The model under review builds one solid part; all positions refer to its coordinate system, in mm. A direction names the side the tool comes from. Coordinates: 2 decimals unless noted, no trailing zeros. Write each loop counter-clockwise with the first axis right and the second up, starting at its lowest first coordinate (ties: lowest second). Pieces come first, ordered by that corner, then holes.
1) Mouldability with a two-part tool opening along X and no side actions: class faces 1 (the flat face through (0, 7.485, 1)), 2 (the flat face through (5.047, 6, 1)), 3 (the cylindrical face through (120, 0, 1)), 4 (the flat face through (54, 0, 3)) as released by +X, released by -X, zero draft, split by the parting line, or undercut.
2) Add section D-D, the plane x = 2.5. State the section outline as (y, z) points.
3) Machinability: for faces 5 (the flat face through (0, 4.985, 1)), 6 (the flat face through (54, -10, 1)), which of the approach directions +Z, -Z, +X, -X, +Y, -Y give a long, thin tool a straight path to every point of the face, cutting with its end or side? Answer none if there is none.
4) Add section A-A, the plane x = 20. State the section outline as (y, z) points.
5) For line 1 (Y direction, x = 0, z = 0.75); line 2 (Y direction, x = 110, z = 2.25); line 3 (Y direction, x = 20, z = 2.1), list the stretches that pass through material, from the lowest coordinate up.
6) Add section C-C, the plane z = 2.5. State the section outline as (x, y) points.
7) Add section B-B, the plane y = 0. State the section outline as (x, z) points, then the cut area to 3 significant figures.
8) For P1, Ø0.8, axis at y = 6.5, z = 1.5, coming from the +X side; P2, Ø0.8, axis at y = 6.5, z = 2, coming from the -X side, all flat-tipped, find the tip position at first contact; note any pin that passes through.
from build123d import *

# Parameters (mm, degrees)
SKETCH1_R           = 4.01
BOSS_EXTRUDE1_DEPTH = 3
CUT_EXTRUDE2_REACH  = 122.453
SKETCH4_W           = 10
SKETCH4_H           = 2.5
SKETCH2_R           = 1.49
CUT_EXTRUDE3_DEPTH  = 10


with BuildPart() as part:
    # Sketch1 → Boss-Extrude1 (new body)
    with BuildSketch(Plane.XY):
        with BuildLine():
            Line((110, 10), (0, 10))
            ThreePointArc((0, 10), (-10, 0), (0, -10))
            Line((0, -10), (110, -10))
            ThreePointArc((110, -10), (120, 0), (110, 10))
        make_face()
        Circle(SKETCH1_R, mode=Mode.SUBTRACT)
        with Locations((110, 0)):
            Circle(SKETCH1_R, mode=Mode.SUBTRACT)
    extrude(amount=BOSS_EXTRUDE1_DEPTH)

    # Sketch4 → Cut-Extrude2 (cut, up to next)
    with BuildSketch(Plane(origin=(0, 0, 0), x_dir=(-1, 0, 0), z_dir=(0, 0, -1)), mode=Mode.PRIVATE) as cut_extrude2_sk1:
        with Locations((-0.046889456, 6.235161972)):
            Rectangle(SKETCH4_W, SKETCH4_H)
    cut_extrude2_tool1 = extrude(cut_extrude2_sk1.sketch, amount=-CUT_EXTRUDE2_REACH, mode=Mode.PRIVATE) & part.part
    add(cut_extrude2_tool1.solids().sort_by_distance((0.046889, 6.235162, 0))[0], mode=Mode.SUBTRACT)

    # Sketch2 → Cut-Extrude3 (cut)
    with BuildSketch(Plane(origin=(0, 0, 0), x_dir=(-1, 0, 0), z_dir=(0, 0, -1))):
        with Locations((-20, 0)):
            Circle(SKETCH2_R)
    extrude(amount=-CUT_EXTRUDE3_DEPTH, mode=Mode.SUBTRACT)


solid = part.part
Geometry results:
1. face 1: undercut
1. face 2: undercut
1. face 3: released by +X
1. face 4: zero draft
2. outline: (-10, 0) - (-3.14, 0) - (-3.14, 3) - (-10, 3) - close; (3.14, 0) - (4.99, 0) - (4.99, 3) - (3.14, 3) - close; (7.49, 0) - (10, 0) - (10, 3) - (7.49, 3) - close
3. face 5: +Z, -Z
3. face 6: +Z, -Z, +X, -X, -Y
4. outline: (-10, 0) - (-1.49, 0) - (-1.49, 3) - (-10, 3) - close; (1.49, 0) - (10, 0) - (10, 3) - (1.49, 3) - close
5. line 1: y = -10 to -4.01, 4.01 to 4.99, 7.49 to 10
5. line 2: y = -10 to -4.01, 4.01 to 10
5. line 3: y = -10 to -1.49, 1.49 to 10
6. outline: (0, -10) - (110, -10) arc R10 ccw to (110, 10) - (0, 10) arc R10 ccw to start; hole (-4.95, 4.99) - (5.05, 4.99) - (5.05, 7.49) - (-4.95, 7.49) - close; hole circle Ø8.02 at (0, 0); hole circle Ø2.98 at (20, 0); hole circle Ø8.02 at (110, 0)
7. outline: (-10, 0) - (-4.01, 0) - (-4.01, 3) - (-10, 3) - close; (4.01, 0) - (18.51, 0) - (18.51, 3) - (4.01, 3) - close; (21.49, 0) - (105.99, 0) - (105.99, 3) - (21.49, 3) - close; (114.01, 0) - (120, 0) - (120, 3) - (114.01, 3) - close
7. area: 333 mm2
8. P1: stops at x = 117.92
8. P2: stops at x = -7.92
